from build123d import *

# Parameters (mm, degrees)
SKETCH1_R           = 1.5875
BOSS_EXTRUDE1_DEPTH = 6.35
SKETCH2_R           = 0.889
CUT_EXTRUDE1_DEPTH  = 6.35


with BuildPart() as part:
    # Sketch1 → Boss-Extrude1 (new body)
    with BuildSketch(Plane.XY):
        with BuildLine():
            Line((-6.193204917, -0.093500134), (12.856795083, -0.093500134))
            Line((12.856795083, -0.093500134), (12.856795083, -5.173500134))
            ThreePointArc((12.856795083, -5.173500134), (12.112846307, -6.969551358), (10.316795083, -7.713500134))
            Line((10.316795083, -7.713500134), (-3.653204917, -7.713500134))
            ThreePointArc((-3.653204917, -7.713500134), (-5.449256142, -6.969551358), (-6.193204917, -5.173500134))
            Line((-6.193204917, -5.173500134), (-6.193204917, -0.093500134))
        make_face()
        with Locations((0.156795083, -3.903500134)):
            Circle(SKETCH1_R, mode=Mode.SUBTRACT)
        with Locations((6.506795083, -3.903500134)):
            Circle(SKETCH1_R, mode=Mode.SUBTRACT)
    extrude(amount=BOSS_EXTRUDE1_DEPTH)

    # Sketch2 → Cut-Extrude1 (cut)
    with BuildSketch(Plane(origin=(0, -0.093500134, 0), x_dir=(1, 0, 0), z_dir=(0, 1, 0))):
        with Locations(Location((-3.811954917, -3.175, 0), (0, 0, 180))):
            Circle(SKETCH2_R)
        with Locations(Location((10.475545083, -3.175, 0), (0, 0, 180))):
            Circle(SKETCH2_R)
    extrude(amount=-CUT_EXTRUDE1_DEPTH, mode=Mode.SUBTRACT)


solid = part.part
CAD build for the part. Positions are in the model's coordinates, mm. A direction names the side the tool comes from. Round coordinates to 2 decimals unless told otherwise and drop trailing zeros. Order: outer loops, then holes, each group sorted by start corner. A loop starts at its lowest first (then second) coordinate and runs counter-clockwise, first axis right, second up. Notation, with made-up numbers: (-27, -10.5) - (24, -10.5) arc R32 ccw to (24, 19.5) - close; hole circle Ø4 at (-29, 56.25). An arc over 180 degrees is marked (long way). Return JSON: item names as keys, results as strings.
(1) Cut at C-C (z = 4.5). Give the cut face in (x, y) (1 decimal).
Answer key:
{"outline": "(-6.2, -5.2) arc R2.5 ccw to (-3.7, -7.7) - (10.3, -7.7) arc R2.5 ccw to (12.9, -5.2) - (12.9, -0.1) - (-6.2, -0.1) - close; hole circle Ø3.2 at (0.2, -3.9); hole circle Ø3.2 at (6.5, -3.9)"}
(2) Wall check: probe 1 along X at (y, z) = (-0.75, 2.75); probe 2 along Y at (x, z) = (0.5, 1.5); probe 3 along X at (y, z) = (-4.5, 3.75). Give the ranges that are in metal, low to high. Write a range as from..to.
Answer key:
{"probe 1": "x = -6.19..-4.59, -3.03..9.69, 11.26..12.86", "probe 2": "y = -7.71..-5.45, -2.35..-0.09", "probe 3": "x = -6.19..-4.49, -3.13..-1.31, 1.63..5.04, 7.98..9.8, 11.15..12.86"}
(3) Cut at D-D (x = 10). Give the cut face in (y, z).
Answer key:
{"outline": "(-7.71, 0) - (-0.09, 0) - (-0.09, 2.42) - (-6.44, 2.42) - (-6.44, 3.93) - (-0.09, 3.93) - (-0.09, 6.35) - (-7.71, 6.35) - close"}
(4) Cut at A-A (y = -2.75). Give the cut face in (x, z) (3 decimals).
Answer key:
{"outline": "(-6.193, 0) - (-0.934, 0) - (-0.934, 6.35) - (-6.193, 6.35) - close; (1.247, 0) - (5.416, 0) - (5.416, 6.35) - (1.247, 6.35) - close; (7.597, 0) - (12.857, 0) - (12.857, 6.35) - (7.597, 6.35) - close; hole circle Ø1.778 at (-3.812, 3.175); hole circle Ø1.778 at (10.476, 3.175)"}
(5) Pin check, flat tip, straight feed: pin 1 Ø2.5 at (x, y) = (6.51, -3.9) entering from -Z. Stop position of the tip, or through.
Answer key:
{"pin 1": "passes through"}
(6) Pull direction Y, two halves, no side cores. Call faces 3 (the face through (9.628, -3.224, 3.442)), 4 (the face through (10, -6.444, 3)), 5 (the face through (-0.187, -5.453, 3.131)): +Y half, -Y half, draft (parallel to the pull), parting line (faces both ways), or undercut.
Answer key:
{"face 3": "draft", "face 4": "+Y half", "face 5": "undercut"}
(7) Cut at B-B (x = -0.25). Give the cut face in (y, z).
Answer key:
{"outline": "(-7.71, 0) - (-5.44, 0) - (-5.44, 6.35) - (-7.71, 6.35) - close; (-2.37, 0) - (-0.09, 0) - (-0.09, 6.35) - (-2.37, 6.35) - close"}
(8) Tool access for faces 1 (the face through (-4, -6.444, 3)), 2 (the face through (-6.193, -3, 3)): list every direction of +Z, -Z, +X, -X, +Y, -Y with a clear straight run to the whole face (end or side of a thin tool).
Answer key:
{"face 1": "+Y", "face 2": "+Z, -Z, -X, +Y, -Y"}
